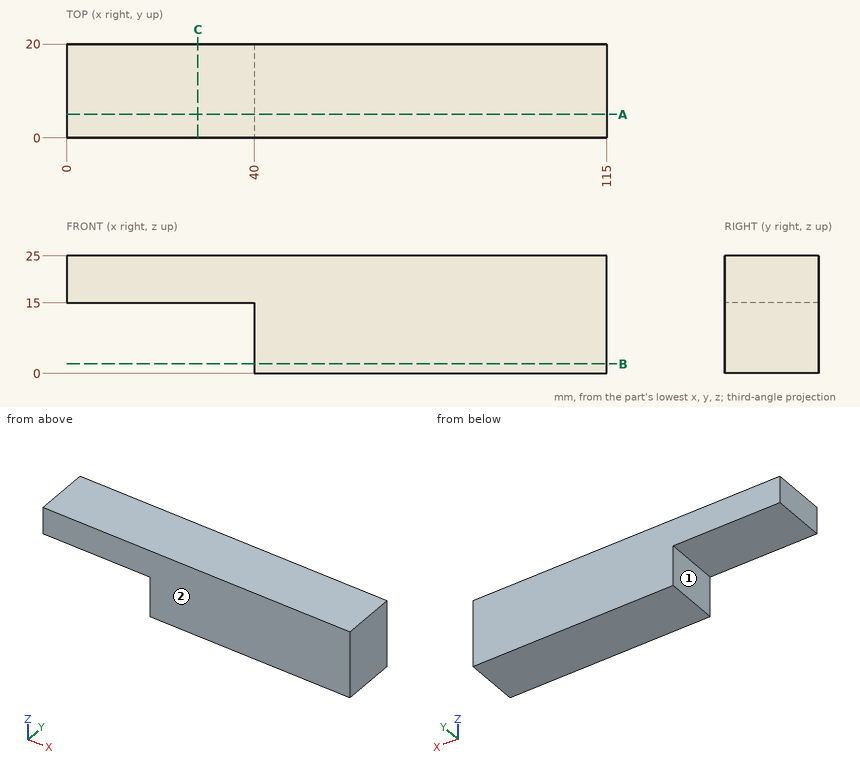
Could you check a few things on this drawing? It's one solid part, dimensions in mm from its lowest x, y, z. A direction names the side the tool comes from. Give positions to 0.01 mm unless a question says otherwise; leave off trailing zeros. Order: outer loops, then holes, each group sorted by start corner. A loop starts at its lowest first (then second) coordinate and runs counter-clockwise, first axis right, second up. Notation, with made-up numbers: (-34.5, 38) - (-27.5, 38) arc R13 cw to (-27.5, 56) - close; hole circle Ø10 at (73, 36). An arc over 180 degrees is marked (long way). Answer as a JSON object with one key per item and string values. Group by question number.
Item 1: If we section it at A-A on y = 5: Please give me the cut outline in (x, z).
Item 2: If we section it at B-B on z = 2: Please give me the cut outline in (x, y), and give its area (3 significant figures).
Item 3: If we section it at C-C on x = 28: Please give me the cut outline in (y, z).
Item 4: Please list where these lines run through material, in increasing order: probe 1 along X at (y, z) = (14, 11.5); probe 2 along Z at (x, y) = (27, 15.25).
Item 5: For P1, Ø6, axis at y = 14.5, z = 15.5, coming from the -X side; P2, Ø5, axis at x = 35.5, z = 7.5, coming from the -Y side; P3, Ø7.5, axis at y = 10.5, z = 10, coming from the -X side, each with a flat end and sliding along its axis, tell me the tip position at first contact or that it passes through.
Item 6: Which directions (+Z, -Z, +X, -X, +Y, -Y) give clear straight access to the entire face, cutting with the end or side of a thin tool? Please do the marked faces 1 and 2.
Result set:
{
 "1": {"outline": "(0, 15) - (40, 15) - (40, 0) - (115, 0) - (115, 25) - (0, 25) - close"},
 "2": {"outline": "(40, 0) - (115, 0) - (115, 20) - (40, 20) - close", "area": "1,500 mm²"},
 "3": {"outline": "(0, 15) - (20, 15) - (20, 25) - (0, 25) - close"},
 "4": {"probe 1": "40 to 115", "probe 2": "15 to 25"},
 "5": {"P1": "x = 0", "P2": "through", "P3": "x = 40"},
 "6": {"face 1": "-Z, -X, +Y, -Y", "face 2": "+Z, -Z, +X, -X, -Y"}
}
